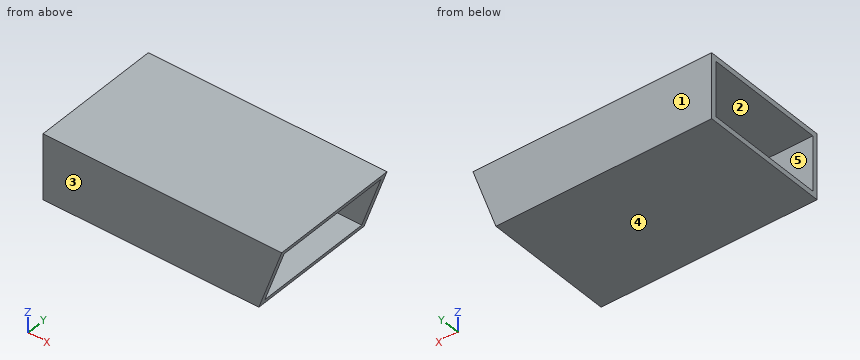
from build123d import *

# Parameters (mm, degrees)
DODANIE_WYCI_GNI_CIE1_DEPTH = 100
SZKIC2_W                    = 42
SZKIC2_H                    = 92
WYTNIJ_WYCI_GNI_CIE1_DEPTH  = 200


with BuildPart() as part:
    # Szkic1 → Dodanie-wyciągnięcie1 (new body)
    with BuildSketch(Plane(origin=(0, 0, 0), x_dir=(1, 0, 0), z_dir=(0, 1, 0))):
        Polygon((0, 0), (182.5, 0), (165, 50), (0, 50), align=None)
    extrude(amount=DODANIE_WYCI_GNI_CIE1_DEPTH)

    # Szkic2 → Wytnij-wyciągnięcie1 (cut)
    with BuildSketch(Plane.ZY):
        with Locations((-25, 50)):
            Rectangle(SZKIC2_W, SZKIC2_H)
    extrude(amount=-WYTNIJ_WYCI_GNI_CIE1_DEPTH, mode=Mode.SUBTRACT)


solid = part.part
Work out the finished part from the listing and answer in its coordinate system (mm). Face numbers are marked on the shaded views. A direction names the side the tool comes from. Give positions to 0.01 mm unless a question says otherwise; leave off trailing zeros. Loops run counter-clockwise (first coordinate to the right, second up) from the corner with the lowest first, then second, coordinate; pieces in that order, holes last. Notation, with made-up numbers: (61, 37) - (72, 37) arc R26 ccw to (72, 74) - close; hole circle Ø6 at (39, 9). An arc over 180 degrees is marked (long way). Answer in a Markdown table with one row per item. Add a question column.
Q1. The part is cut by section A-A (z = -21). Determine the outline of the cut face in (x, y), and give its area (3 significant figures).
Q2. A tool of negligible diameter and unlimited length cuts with its end or side. For the marked faces 1 and 2, from which of +Z, -Z, +X, -X, +Y, -Y can it reach the whole face along a straight path? Write none if from no direction.
Q3. Consider line 1 along Y through (x, z) = (106, -11.5); line 2 along Z through (x, y) = (77, 60); line 3 along Z through (x, y) = (168.5, 27). Determine where each line is inside the solid, lowest interval first.
Q4. This flat-tipped pin is pushed along its axis until it touches: P1, Ø4, axis at x = 71, y = 66, coming from the +Z side. Where does it stop, or does it pass through?
Q5. The part is cut by section B-B (y = 26.5). Determine the outline of the cut face in (x, z), and give its area (3 significant figures).
Q6. The part is cut by section C-C (x = 31). Determine the outline of the cut face in (y, z).
Q7. Determine the mould class of the marked faces 3, 4 and 5 for opening direction Y: released by +Y, released by -Y, zero draft, split by the parting line, or undercut.
Solution:
| question | item | result |
|---|---|---|
| 1 | outline | (0, 0) - (175.15, 0) - (175.15, 4) - (0, 4) - close; (0, 96) - (175.15, 96) - (175.15, 100) - (0, 100) - close |
| 1 | area | 1,400 mm² |
| 2 | face 1 | +Z, -Z, +X, -X, +Y |
| 2 | face 2 | +X, -X |
| 3 | line 1 | y = 0 to 4, 96 to 100 |
| 3 | line 2 | z = -50 to -46, -4 to 0 |
| 3 | line 3 | z = -4 to 0 |
| 4 | P1 | stops at z = 0 |
| 5 | outline | (0, -50) - (165, -50) - (166.4, -46) - (0, -46) - close; (0, -4) - (181.1, -4) - (182.5, 0) - (0, 0) - close |
| 5 | area | 1,390 mm² |
| 6 | outline | (0, -50) - (100, -50) - (100, 0) - (0, 0) - close; hole (4, -46) - (96, -46) - (96, -4) - (4, -4) - close |
| 7 | face 3 | released by -Y |
| 7 | face 4 | zero draft |
| 7 | face 5 | undercut |
